```python
from build123d import *

# Parameters (mm, degrees)
SKETCH1_W           = 46.539672572
SKETCH1_H           = 19.211338676
SKETCH1_H_2         = 18.276713521
SKETCH1_H_3         = 18.27671352
BOSS_EXTRUDE1_DEPTH = 5


with BuildPart() as part:
    # Sketch1 → Boss-Extrude1 (new body)
    with BuildSketch(Plane(origin=(0, 0, 0), x_dir=(1, 0, 0), z_dir=(0, 1, 0))):
        Polygon((-14.77881137, 25.162411855), (14.42118863, 25.162411855), (14.42118863, 30.433230433), (34.42118863, 30.433230433), (34.42118863, 25.433230433), (34.42118863, -90.566769567), (34.42118863, -95.566769567), (14.42118863, -95.566769567), (14.42118863, -90.29595099), (-14.77881137, -90.29595099), (-14.77881137, -95.566769567), (-34.77881137, -95.566769567), (-34.77881137, -90.566769567), (-34.77881137, 25.433230433), (-34.77881137, 30.433230433), (-14.77881137, 30.433230433), align=None)
        with Locations((0.760939105, -46.129253173)):
            Rectangle(SKETCH1_W, SKETCH1_H, mode=Mode.SUBTRACT)
        with Locations((0.760939105, 6.711270036)):
            Rectangle(SKETCH1_W, SKETCH1_H_2, mode=Mode.SUBTRACT)
        with Locations((0.760939105, -19.004285962)):
            Rectangle(SKETCH1_W, SKETCH1_H, mode=Mode.SUBTRACT)
        with Locations((0.760939105, -71.84480917)):
            Rectangle(SKETCH1_W, SKETCH1_H_3, mode=Mode.SUBTRACT)
    extrude(amount=BOSS_EXTRUDE1_DEPTH)


solid = part.part
```
Model file for the job. Use its own axes, mm. A direction names the side the tool comes from. Coordinates: 2 decimals unless noted, no trailing zeros. Write each loop counter-clockwise with the first axis right and the second up, starting at its lowest first coordinate (ties: lowest second). Pieces come first, ordered by that corner, then holes. Notation, with made-up numbers: (-4, 42) - (1, 42) arc R23 cw to (1, 60) - close; hole circle Ø9 at (80.25, 13). An arc over 180 degrees is marked (long way). One line per item, written item: value. Start each with the question number.
1. Slice it at C-C (y = 2.1). Write the cut outline in (x, z), plus the area to 3 significant figures.
2. Mould opens along Z. For faces 5 (the flat face through (-14.779, 2, 93)), 6 (the flat face through (25, 2, 95.567)), 7 (the flat face through (0, 2, 55.735)) say: released by +Z, released by -Z, zero draft, split by the parting line, or undercut.
3. Tool access for faces 1 (the flat face through (0, 2, -25.162)), 2 (the flat face through (0, 2, 62.706)), 3 (the flat face through (-34.779, 2, 32)), 4 (the flat face through (14.421, 2, 93)): list every direction of +Z, -Z, +X, -X, +Y, -Y with a clear straight run to the whole face (end or side of a thin tool).
4. Slice it at A-A (z = 72.5). Write the cut outline in (x, y).
5. Slice it at B-B (x = -9). Write the cut outline in (y, z), plus the area to 3 significant figures.
6. Flat gauge pins, fed straight in: pin 1 (1.5 mm diameter, centred on x = 8.5, y = 3, fed in from +Z); pin 2 (2.5 mm diameter, centred on x = -1, y = 2.5, fed in from -Z). Where does each tip first touch, or does it go through?
7. Slice it at D-D (x = -18). Write the cut outline in (y, z).
8. Probe line 1 (Z direction, x = 10, y = 2.8); line 2 (Z direction, x = 15, y = 4.5); line 3 (X direction, y = 4.5, z = 9.5). List the from-to ranges inside material, lowest first. Write a range as from..to.
Answers below:
1. outline: (-34.78, -30.43) - (-14.78, -30.43) - (-14.78, -25.16) - (14.42, -25.16) - (14.42, -30.43) - (34.42, -30.43) - (34.42, 95.57) - (14.42, 95.57) - (14.42, 90.3) - (-14.78, 90.3) - (-14.78, 95.57) - (-34.78, 95.57) - close; hole (-22.51, -15.85) - (24.03, -15.85) - (24.03, 2.43) - (-22.51, 2.43) - close; hole (-22.51, 9.4) - (24.03, 9.4) - (24.03, 28.61) - (-22.51, 28.61) - close; hole (-22.51, 36.52) - (24.03, 36.52) - (24.03, 55.73) - (-22.51, 55.73) - close; hole (-22.51, 62.71) - (24.03, 62.71) - (24.03, 80.98) - (-22.51, 80.98) - close
1. area: 4,920 mm^2
2. face 5: zero draft
2. face 6: released by +Z
2. face 7: undercut
3. face 1: -Z, +Y, -Y
3. face 2: +Y, -Y
3. face 3: +Z, -Z, -X, +Y, -Y
3. face 4: +Z, +Y, -Y
4. outline: (-34.78, 0) - (-22.51, 0) - (-22.51, 5) - (-34.78, 5) - close; (24.03, 0) - (34.42, 0) - (34.42, 5) - (24.03, 5) - close
5. outline: (0, -25.16) - (5, -25.16) - (5, -15.85) - (0, -15.85) - close; (0, 2.43) - (5, 2.43) - (5, 9.4) - (0, 9.4) - close; (0, 28.61) - (5, 28.61) - (5, 36.52) - (0, 36.52) - close; (0, 55.73) - (5, 55.73) - (5, 62.71) - (0, 62.71) - close; (0, 80.98) - (5, 80.98) - (5, 90.3) - (0, 90.3) - close
5. area: 202 mm^2
6. pin 1: stops at z = 90.3
6. pin 2: stops at z = -25.16
7. outline: (0, -30.43) - (5, -30.43) - (5, -15.85) - (0, -15.85) - close; (0, 2.43) - (5, 2.43) - (5, 9.4) - (0, 9.4) - close; (0, 28.61) - (5, 28.61) - (5, 36.52) - (0, 36.52) - close; (0, 55.73) - (5, 55.73) - (5, 62.71) - (0, 62.71) - close; (0, 80.98) - (5, 80.98) - (5, 95.57) - (0, 95.57) - close
8. line 1: z = -25.16..-15.85, 2.43..9.4, 28.61..36.52, 55.73..62.71, 80.98..90.3
8. line 2: z = -30.43..-15.85, 2.43..9.4, 28.61..36.52, 55.73..62.71, 80.98..95.57
8. line 3: x = -34.78..-22.51, 24.03..34.42
